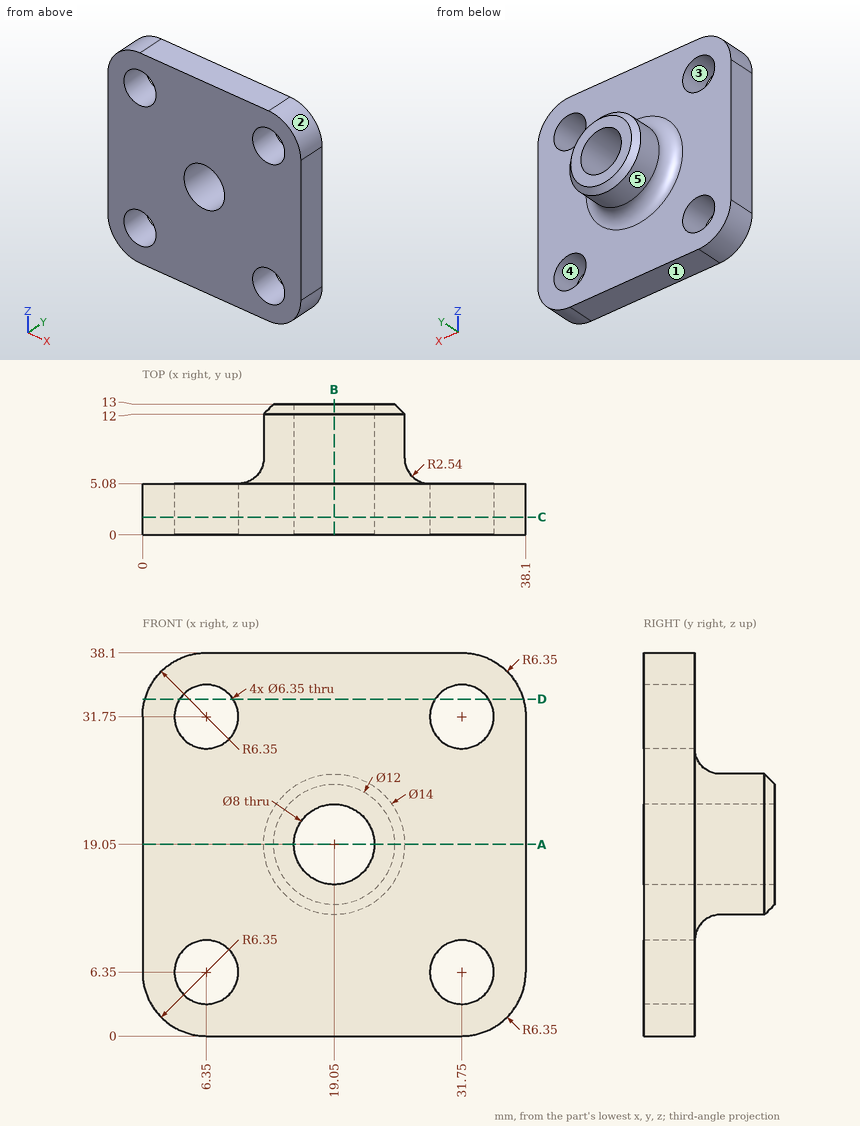
Study the drawing (mm; zero at the part's minimum x, y, z) and answer. A direction names the side the tool comes from. Round coordinates to 2 decimals unless told otherwise and drop trailing zeros. Loops run counter-clockwise (first coordinate to the right, second up) from the corner with the lowest first, then second, coordinate; pieces in that order, holes last.
Q1. Section D-D, the plane z = 33.5 is taken. Determine the outline of the cut face in (x, y), then the cut area to 3 significant figures.
Q2. Which of the six approach directions +Z, -Z, +X, -X, +Y, -Y give full straight-line access (tool end or side, diameter ignored) to the marked faces 4 and 5?
Q3. Find the intervals of material crossed by line 1 (X direction, y = 3.25, z = 32); line 2 (Z direction, x = 30, y = 1.75); line 3 (Y direction, x = 19, z = 36.5), in increasing order.
Q4. Section C-C, the plane y = 1.75 is taken. Determine the outline of the cut face in (x, z) (3 decimals).
Q5. For a pull along X with two mould halves and no side action, classify the marked faces 1, 2 and 3 as released by +X, released by -X, zero draft, split by the parting line, or undercut.
Q6. Given pin 1 Ø7.5 at (x, z) = (31.75, 6.35) entering from +Y; pin 2 Ø5 at (y, z) = (9, 7) entering from +X; pin 3 Ø2 at (x, y) = (14.5, 8) entering from +Z, each flat-ended and moving along its own axis, determine where each tip first touches the part or whether it passes through.
Q7. Section A-A, the plane z = 19.05 is taken. Determine the outline of the cut face in (x, y), then the cut area to 3 significant figures.
Q8. Section B-B, the plane x = 19.05 is taken. Determine the outline of the cut face in (y, z), then the cut area to 3 significant figures.
Completed:
1. outline: (0.25, 0) - (3.7, 0) - (3.7, 5.08) - (0.25, 5.08) - close; (9, 0) - (29.1, 0) - (29.1, 5.08) - (9, 5.08) - close; (34.4, 0) - (37.85, 0) - (37.85, 5.08) - (34.4, 5.08) - close
1. area: 137 mm2
2. face 4: +Y, -Y
2. face 5: +Y
3. line 1: x = 0 to 3.18, 9.52 to 28.58, 34.92 to 38.1
3. line 2: z = 0 to 3.7, 9 to 29.1, 34.4 to 38.1
3. line 3: y = 0 to 5.08
4. outline: (0, 6.35) arc R6.35 ccw to (6.35, 0) - (31.75, 0) arc R6.35 ccw to (38.1, 6.35) - (38.1, 31.75) arc R6.35 ccw to (31.75, 38.1) - (6.35, 38.1) arc R6.35 ccw to (0, 31.75) - close; hole circle Ø6.35 at (6.35, 6.35); hole circle Ø6.35 at (6.35, 31.75); hole circle Ø8 at (19.05, 19.05); hole circle Ø6.35 at (31.75, 6.35); hole circle Ø6.35 at (31.75, 31.75)
5. face 1: zero draft
5. face 2: released by +X
5. face 3: undercut
6. pin 1: stops at y = 5.08
6. pin 2: passes through
6. pin 3: stops at z = 25.08
7. outline: (0, 0) - (15.05, 0) - (15.05, 13) - (13.05, 13) - (12.05, 12) - (12.05, 7.62) arc R2.54 cw to (9.51, 5.08) - (0, 5.08) - close; (23.05, 0) - (38.1, 0) - (38.1, 5.08) - (28.59, 5.08) arc R2.54 cw to (26.05, 7.62) - (26.05, 12) - (25.05, 13) - (23.05, 13) - close
7. area: 202 mm2
8. outline: (0, 0) - (5.08, 0) - (5.08, 9.51) arc R2.54 cw to (7.62, 12.05) - (12, 12.05) - (13, 13.05) - (13, 15.05) - (0, 15.05) - close; (0, 23.05) - (13, 23.05) - (13, 25.05) - (12, 26.05) - (7.62, 26.05) arc R2.54 cw to (5.08, 28.59) - (5.08, 38.1) - (0, 38.1) - close
8. area: 202 mm2
